from build123d import *

# Parameters (mm, degrees)
BOSS_EXTRUDE1_DEPTH = 50
SKETCH2_R           = 2.5
CUT_EXTRUDE1_DEPTH  = 100
CHAMFER1_SIZE       = 3
SKETCH3_R           = 2.6
CUT_EXTRUDE2_DEPTH  = 93.741576437
SKETCH6_R           = 5.5
CUT_EXTRUDE3_DEPTH  = 93.741576437
SKETCH7_W           = 74
SKETCH7_H           = 5
BOSS_EXTRUDE2_DEPTH = 20
FILLET1_R           = 4
SKETCH8_W           = 34
SKETCH8_H           = 6.5
BOSS_EXTRUDE3_DEPTH = 5
SKETCH9_R           = 2.75
CUT_EXTRUDE4_DEPTH  = 97.401504138
CHAMFER2_SIZE       = 3
FILLET2_R           = 4


with BuildPart() as part:
    # Sketch1 → Boss-Extrude1 (new body)
    with BuildSketch(Plane.XY):
        Polygon((0, 0), (0, 25), (74, 25), (74, 0), (69, 0), (69, 20), (5, 20), (5, 0), align=None)
    extrude(amount=BOSS_EXTRUDE1_DEPTH)

    # Sketch2 → Cut-Extrude1 (cut, symmetric)
    with BuildSketch(Plane(origin=(5, 0, 0), x_dir=(0, 0, -1), z_dir=(1, 0, 0))):
        with Locations((-42, 10)):
            Circle(SKETCH2_R)
        with Locations((-8, 10)):
            Circle(SKETCH2_R)
    extrude(amount=CUT_EXTRUDE1_DEPTH, both=True, mode=Mode.SUBTRACT)

    # Chamfer1
    chamfer1_edges = [part.edges().sort_by_distance(p)[0] for p in [
        (2.5, 0, 0),
        (71.5, 0, 50),
        (2.5, 0, 50),
        (71.5, 0, 0),
    ]]
    chamfer(chamfer1_edges, length=CHAMFER1_SIZE)

    # Sketch3 → Cut-Extrude2 (cut, through all)
    with BuildSketch(Plane(origin=(0, 25, 0), x_dir=(1, 0, 0), z_dir=(0, 1, 0))):
        with Locations(Location((11.5, -45, 0), (0, 0, 180))):
            Circle(SKETCH3_R)
        with Locations(Location((62.5, -45, 0), (0, 0, 180))):
            Circle(SKETCH3_R)
        with Locations(Location((62.5, -5, 0), (0, 0, 180))):
            Circle(SKETCH3_R)
        with Locations(Location((11.5, -5, 0), (0, 0, 180))):
            Circle(SKETCH3_R)
    extrude(amount=-CUT_EXTRUDE2_DEPTH, mode=Mode.SUBTRACT)

    # Sketch6 → Cut-Extrude3 (cut, through all)
    with BuildSketch(Plane(origin=(0, 25, 0), x_dir=(1, 0, 0), z_dir=(0, 1, 0))):
        with Locations(Location((37, -37.5, 0), (0, 0, 180))):
            Circle(SKETCH6_R)
        with Locations(Location((37, -12.5, 0), (0, 0, 180))):
            Circle(SKETCH6_R)
    extrude(amount=-CUT_EXTRUDE3_DEPTH, mode=Mode.SUBTRACT)

    # Sketch7 → Boss-Extrude2 (add)
    with BuildSketch(Plane.XZ):
        with Locations((37, 25)):
            Rectangle(SKETCH7_W, SKETCH7_H)
    extrude(amount=-BOSS_EXTRUDE2_DEPTH)

    # Fillet1
    fillet1_edges = [part.edges().sort_by_distance(p)[0] for p in [
        (5, 10, 22.5),
        (5, 10, 27.5),
        (69, 10, 22.5),
        (69, 10, 27.5),
    ]]
    fillet(fillet1_edges, radius=FILLET1_R)

    # Sketch8 → Boss-Extrude3 (add)
    with BuildSketch(Plane(origin=(0, 25, 0), x_dir=(1, 0, 0), z_dir=(0, 1, 0))):
        with Locations((37, 3.25)):
            Rectangle(SKETCH8_W, SKETCH8_H)
    boss_extrude3 = extrude(amount=-BOSS_EXTRUDE3_DEPTH)

    # Mirror1: Boss-Extrude3 across plane
    add(boss_extrude3.mirror(Plane.XY.offset(25)))

    # Sketch9 → Cut-Extrude4 (cut, through all)
    with BuildSketch(Plane(origin=(0, 25, 0), x_dir=(1, 0, 0), z_dir=(0, 1, 0))):
        with Locations(Location((27, 0.5, 0), (0, 0, 180))):
            Circle(SKETCH9_R)
        with Locations(Location((47, 0.5, 0), (0, 0, 180))):
            Circle(SKETCH9_R)
        with Locations(Location((27, -50.5, 0), (0, 0, 180))):
            Circle(SKETCH9_R)
        with Locations(Location((47, -50.5, 0), (0, 0, 180))):
            Circle(SKETCH9_R)
    extrude(amount=-CUT_EXTRUDE4_DEPTH, mode=Mode.SUBTRACT)

    # Chamfer2
    chamfer2_edges = [part.edges().sort_by_distance(p)[0] for p in [
        (20, 22.5, -6.5),
        (54, 22.5, -6.5),
        (20, 22.5, 56.5),
        (54, 22.5, 56.5),
    ]]
    chamfer(chamfer2_edges, length=CHAMFER2_SIZE)

    # Fillet2
    # the kernel refuses this fillet: 4 mm, written as the material it adds along each edge
    with BuildSketch(Plane(origin=(20, 25, 50), x_dir=(-1, 0, 0), z_dir=(0, -1, 0))) as fillet2_piece_1:
        with BuildLine():
            CenterArc((3.968626967, -4), FILLET2_R, 90, 82.819244219)
            Line((0, -3.5), (-0.079372539, -3.49))
            ThreePointArc((-0.079372539, -3.49), (-0.08, -1.75), (-0.08, 0))
            Line((-0.08, 0), (0, 0.08))
            Line((0, 0.08), (3.968626967, 0.08))
            Line((3.968626967, 0.08), (3.968626967, 0))
        make_face()
    extrude(amount=5)
    with BuildSketch(Plane(origin=(54, 25, 50), x_dir=(1, 0, 0), z_dir=(0, -1, 0))) as fillet2_piece_2:
        with BuildLine():
            CenterArc((3.968626967, 4), FILLET2_R, 187.180755781, 82.819244219)
            Line((0, 3.5), (-0.079372539, 3.49))
            ThreePointArc((-0.079372539, 3.49), (-0.08, 1.75), (-0.08, 0))
            Line((-0.08, 0), (0, -0.08))
            Line((0, -0.08), (3.968626967, -0.08))
            Line((3.968626967, -0.08), (3.968626967, 0))
        make_face()
    extrude(amount=5)
    with BuildSketch(Plane(origin=(54, 25, 0), x_dir=(0, 0, -1), z_dir=(0, -1, 0))) as fillet2_piece_3:
        with BuildLine():
            CenterArc((4, 3.968626967), FILLET2_R, 180, 82.819244219)
            Line((0, 3.968626967), (-0.08, 3.968626967))
            Line((-0.08, 3.968626967), (-0.08, 0))
            Line((-0.08, 0), (0, -0.08))
            ThreePointArc((0, -0.08), (1.75, -0.08), (3.49, -0.079372539))
            Line((3.49, -0.079372539), (3.5, 0))
        make_face()
    extrude(amount=5)
    with BuildSketch(Plane(origin=(20, 25, 0), x_dir=(0, 0, -1), z_dir=(0, -1, 0))) as fillet2_piece_4:
        with BuildLine():
            CenterArc((4, -3.968626967), FILLET2_R, 97.180755781, 82.819244219)
            Line((0, -3.968626967), (-0.08, -3.968626967))
            Line((-0.08, -3.968626967), (-0.08, 0))
            Line((-0.08, 0), (0, 0.08))
            ThreePointArc((0, 0.08), (1.75, 0.08), (3.49, 0.079372539))
            Line((3.49, 0.079372539), (3.5, 0))
        make_face()
    extrude(amount=5)


solid = part.part
For this review, take the finished solid that the model builds, in its own axes (mm). A direction names the side the tool comes from. Give positions to 0.01 mm unless a question says otherwise; leave off trailing zeros. Order: outer loops, then holes, each group sorted by start corner. A loop starts at its lowest first (then second) coordinate and runs counter-clockwise, first axis right, second up. Notation, with made-up numbers: (66.25, 31) - (93.25, 31) arc R11 cw to (93.25, 44) - close; hole circle Ø7 at (70, -31). An arc over 180 degrees is marked (long way). Answer as a JSON object with one key per item and string values. Group by question number.
Item 1: Take a section at B-B on x = 27. Give the boundary of the cut face in (y, z).
Item 2: Take a section at D-D on z = 40.5. Give the boundary of the cut face in (x, y).
Item 3: Machinability: for faces 1 (the flat face through (37, 20, 45)), 2 (the cylindrical face through (6.141, 10.14, 21.297)), 3 (the flat face through (4.6, 16.6, 50)), which of the approach directions +Z, -Z, +X, -X, +Y, -Y give a long, thin tool a straight path to every point of the face, cutting with its end or side? Answer none if there is none.
Item 4: Take a section at C-C on y = 15.75. Give the boundary of the cut face in (x, z).
Item 5: Clearance check with flat-ended pins moving along their axes: pin 1 Ø17.5 at (x, z) = (37, 37.5) entering from -Y; pin 2 Ø1.5 at (x, y) = (38, 10.5) entering from +Z; pin 3 Ø10 at (x, y) = (49, 9) entering from -Z; pin 4 Ø4 at (y, z) = (10, 8) entering from +X. State where each tip first meets the part, or that it passes through.
Item 6: Wall thickness on line 1 along Z through (x, y) = (37, 23.5); line 2 along Z through (x, y) = (62.5, 23.15); line 3 along X through (y, z) = (1.5, 36.5): over which ranges is each line inside the solid? List them lowest first.
Item 7: Draft analysis for pull direction Z (two halves, no side actions). For faces 4 (the flat face through (37, 10, 22.5)), 5 (the cylindrical face through (2.54, 9.04, 39.69)), 6 (the cylindrical face through (6.141, 10.14, 28.703)), state which applies: pulls with the +Z half, pulls with the -Z half, needs draft (parallel to the pull), parting line crosses it, or undercut.
Item 8: Take a section at A-A on z = 12.5. Give the boundary of the cut face in (x, y), and give its area (3 significant figures).
Reported:
{
 "1": {"outline": "(0, 22.5) - (20, 22.5) - (20, 2.25) - (25, 2.25) - (25, 47.75) - (20, 47.75) - (20, 27.5) - (0, 27.5) - close; (20, -6.5) - (25, -6.5) - (25, -3.25) - (20, -3.25) - close; (20, 53.25) - (25, 53.25) - (25, 56.5) - (20, 56.5) - close"},
 "2": {"outline": "(0, 0) - (5, 0) - (5, 8) - (0, 8) - close; (0, 12) - (5, 12) - (5, 20) - (32.39, 20) - (32.39, 25) - (0, 25) - close; (41.61, 20) - (69, 20) - (69, 12) - (74, 12) - (74, 25) - (41.61, 25) - close; (69, 0) - (74, 0) - (74, 8) - (69, 8) - close"},
 "3": {"face 1": "+Z, -Y", "face 2": "-Z, -Y", "face 3": "+Z, -X, +Y, -Y"},
 "4": {"outline": "(0, 0) - (5, 0) - (5, 18.5) arc R4 cw to (9, 22.5) - (65, 22.5) arc R4 cw to (69, 18.5) - (69, 0) - (74, 0) - (74, 50) - (69, 50) - (69, 31.5) arc R4 cw to (65, 27.5) - (9, 27.5) arc R4 cw to (5, 31.5) - (5, 50) - (0, 50) - close"},
 "5": {"pin 1": "y = 20", "pin 2": "z = 27.5", "pin 3": "z = 22.5", "pin 4": "through"},
 "6": {"line 1": "-6.5 to 7, 18 to 32, 43 to 56.5", "line 2": "0 to 2.4, 7.6 to 42.4, 47.6 to 50", "line 3": "0 to 5, 69 to 74"},
 "7": {"face 4": "pulls with the -Z half", "face 5": "undercut", "face 6": "pulls with the +Z half"},
 "8": {"outline": "(0, 0) - (5, 0) - (5, 20) - (31.5, 20) - (31.5, 25) - (0, 25) - close; (42.5, 20) - (69, 20) - (69, 0) - (74, 0) - (74, 25) - (42.5, 25) - close", "area": "515 mm^2"}
}
